Read the model definition and answer for the solid it produces. Units are mm, in the model's axes. A direction names the side the tool comes from. Coordinates: 2 decimals unless noted, no trailing zeros. Write each loop counter-clockwise with the first axis right and the second up, starting at its lowest first coordinate (ties: lowest second). Pieces come first, ordered by that corner, then holes. Notation, with made-up numbers: (54, -16.5) -> (72, -16.5) arc R31 cw to (72, 20.5) -> close; hole circle Ø8 at (-21.75, 51). An arc over 180 degrees is marked (long way). Return JSON: item names as keys, results as strings.
from build123d import *

# Parameters (mm, degrees)
SKETCH1_W           = 8
SKETCH1_H           = 9
BOSS_EXTRUDE1_DEPTH = 1
SKETCH6_R           = 4
BOSS_EXTRUDE2_DEPTH = 1
SKETCH9_R           = 4
BOSS_EXTRUDE3_DEPTH = 1


with BuildPart() as part:
    # Sketch1 → Boss-Extrude1 (new body)
    with BuildSketch(Plane(origin=(0, 0, 0), x_dir=(1, 0, 0), z_dir=(0, 1, 0))):
        Rectangle(SKETCH1_W, SKETCH1_H)
    extrude(amount=BOSS_EXTRUDE1_DEPTH)

    # Sketch6 → Boss-Extrude2 (add)
    with BuildSketch(Plane.ZY.offset(-4)):
        with BuildLine():
            Line((4.5, 1), (4.5, -19.5))
            ThreePointArc((4.5, -19.5), (0, -24), (-4.5, -19.5))
            Line((-4.5, -19.5), (-4.5, 1))
            Line((-4.5, 1), (4.5, 1))
        make_face()
        with Locations((0, -19.5)):
            Circle(SKETCH6_R, mode=Mode.SUBTRACT)
    extrude(amount=BOSS_EXTRUDE2_DEPTH)

    # Sketch9 → Boss-Extrude3 (add)
    with BuildSketch(Plane(origin=(-4, 0, 0), x_dir=(0, 0, -1), z_dir=(1, 0, 0))):
        with BuildLine():
            Line((-4.5, 1), (-4.5, -19.5))
            ThreePointArc((-4.5, -19.5), (0, -24), (4.5, -19.5))
            Line((4.5, -19.5), (4.5, 1))
            Line((4.5, 1), (-4.5, 1))
        make_face()
        with Locations(Location((0, -19.5, 0), (0, 0, 180))):
            Circle(SKETCH9_R, mode=Mode.SUBTRACT)
    extrude(amount=-BOSS_EXTRUDE3_DEPTH)


solid = part.part
1. For a pull along Y with two mould halves and no side action, classify faces 1 (the face through (4, -9, 0)), 2 (the face through (-1, 0, 0)), 3 (the face through (0, 1, 0)), 4 (the face through (-4.493, -23.466, -0.521)) as +Y half, -Y half, draft (parallel to the pull), parting line (faces both ways), or undercut.
Taken from the geometry:
{"face 1": "draft", "face 2": "-Y half", "face 3": "+Y half", "face 4": "undercut"}
2. The part is cut by section A-A (y = -1). Determine the outline of the cut face in (x, z), then the cut area to 3 significant figures.
Taken from the geometry:
{"outline": "(-5, -4.5) -> (-4, -4.5) -> (-4, 4.5) -> (-5, 4.5) -> close; (3, -4.5) -> (4, -4.5) -> (4, 4.5) -> (3, 4.5) -> close", "area": "18.0 mm2"}
3. Consider L1, parallel to Y at x = -4.2, z = 0; L2, parallel to X at y = -0.75, z = 0.5; L3, parallel to Z at x = -4.45, y = -19.5. Determine where each line is inside the solid, lowest interval first.
Taken from the geometry:
{"L1": "y = -24 to -23.5, -15.5 to 1", "L2": "x = -5 to -4, 3 to 4", "L3": "z = -4.5 to -4, 4 to 4.5"}
4. The part is cut by section C-C (y = -18.75). Determine the outline of the cut face in (x, z), then the cut area to 3 significant figures.
Taken from the geometry:
{"outline": "(-5, -4.5) -> (-4, -4.5) -> (-4, -3.93) -> (-5, -3.93) -> close; (-5, 3.93) -> (-4, 3.93) -> (-4, 4.5) -> (-5, 4.5) -> close; (3, -4.5) -> (4, -4.5) -> (4, -3.93) -> (3, -3.93) -> close; (3, 3.93) -> (4, 3.93) -> (4, 4.5) -> (3, 4.5) -> close", "area": "2.28 mm2"}
5. The part is cut by section B-B (z = 0). Determine the outline of the cut face in (x, y), then the cut area to 3 significant figures.
Taken from the geometry:
{"outline": "(-5, -24) -> (-4, -24) -> (-4, -23.5) -> (-5, -23.5) -> close; (-5, -15.5) -> (-4, -15.5) -> (-4, 0) -> (3, 0) -> (3, -15.5) -> (4, -15.5) -> (4, 1) -> (-5, 1) -> close; (3, -24) -> (4, -24) -> (4, -23.5) -> (3, -23.5) -> close", "area": "41.0 mm2"}
6. A tool of negligible diameter and unlimited length cuts with its end or side. For faces 5 (the face through (-4.15, -7.78, -4.5)), 6 (the face through (-4, -9, 0)), from which of +Z, -Z, +X, -X, +Y, -Y can it reach the whole face along a straight path? Write none if from no direction.
Taken from the geometry:
{"face 5": "-Z, +X, -X, +Y, -Y", "face 6": "+Z, -Z, -Y"}
7. Flat-ended cylindrical pins translate along their axes: pin 1 Ø4 at (x, y) = (-1.5, -20.5) entering from +Z; pin 2 Ø4 at (y, z) = (-19.5, -2.5) entering from -X. Find the tip coordinate at first contact, or state that the pin passes through.
Taken from the geometry:
{"pin 1": "passes through", "pin 2": "stops at x = -5"}
8. The part is cut by section D-D (z = -3.75). Determine the outline of the cut face in (x, y).
Taken from the geometry:
{"outline": "(-5, -21.99) -> (-4, -21.99) -> (-4, -20.89) -> (-5, -20.89) -> close; (-5, -18.11) -> (-4, -18.11) -> (-4, 0) -> (3, 0) -> (3, -18.11) -> (4, -18.11) -> (4, 1) -> (-5, 1) -> close; (3, -21.99) -> (4, -21.99) -> (4, -20.89) -> (3, -20.89) -> close"}
